Job drawing, mm, ordinate dimensions from the low corner. One solid piece. Coordinates: 2 decimals unless noted, no trailing zeros. Loops run counter-clockwise (first coordinate to the right, second up) from the corner with the lowest first, then second, coordinate; pieces in that order, holes last. Notation, with made-up numbers: (-6.5, -17) -> (16.5, -17) arc R31 ccw to (16.5, 10) -> close; hole circle Ø3 at (54.25, -32.5). An arc over 180 degrees is marked (long way). Use one line per item in the form item = value. Start each with the question number.
(1) Drill centre lines: L1, parallel to Y at x = 6, z = 24.5; L2, parallel to X at y = 4.25, z = 23.5; L3, parallel to X at y = 6.5, z = 36. Where is each one in solid material? Low to high. Write a range as [from, to].
(2) Band-saw the part on A-A on z = 29. Give the cut face in (x, y).
(3) Pin check, flat tips, straight feed: P1, Ø5, axis at y = 3, z = 29.5, coming from the -X side; P2, Ø2, axis at y = 9, z = 26.5, coming from the -X side; P3, Ø4, axis at x = 6, y = 6, coming from the +Z side. Stop position of each tip, or through.
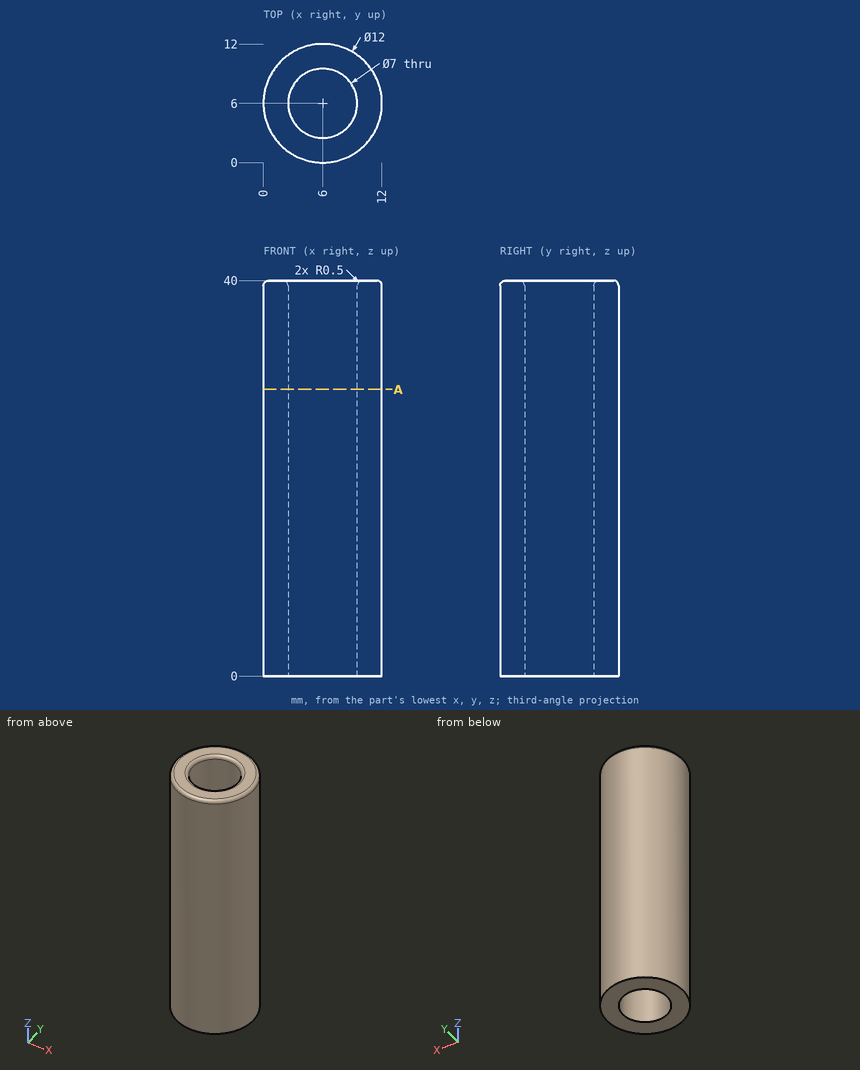
A:
q1.L1 = [0, 2.5], [9.5, 12]
q1.L2 = [0.26, 2.97], [9.03, 11.74]
q1.L3 = [0.02, 2.54], [9.46, 11.98]
q2.outline = circle Ø12 at (6, 6); hole circle Ø7 at (6, 6)
q3.P1 = 0.02
q3.P2 = 0.34
q3.P3 = through
